from build123d import *

# Parameters (mm, degrees)
BOSS_EXTRU_1_DEPTH      = 10
ESQUISSE2_W             = 42
ESQUISSE2_H             = 42
BOSS_EXTRU_2_DEPTH      = 10
ESQUISSE3_W             = 42
ESQUISSE3_H             = 42
BOSS_EXTRU_3_DEPTH      = 10
ESQUISSE4_R             = 11
BOSS_EXTRU_4_DEPTH      = 3
CONG_1_R                = 0.5
ESQUISSE5_R             = 5
ENL_V_MAT_EXTRU_1_DEPTH = 10
ESQUISSE6_R             = 2.5
BOSS_EXTRU_5_DEPTH      = 30
ENL_V_MAT_EXTRU_2_DEPTH = 20
CHANFREIN1_SIZE         = 0.5
ESQUISSE8_R             = 1.5
ENL_V_MAT_EXTRU_3_DEPTH = 5
ENL_V_MAT_EXTRU_5_DEPTH = 41
ESQUISSE11_W            = 5
ESQUISSE11_H            = 10
ENL_V_MAT_EXTRU_6_DEPTH = 3


with BuildPart() as part:
    # Esquisse1 → Boss.-Extru.1 (new body, symmetric)
    with BuildSketch(Plane(origin=(0, 0, 0), x_dir=(0, 0, -1), z_dir=(1, 0, 0))):
        Polygon((6, 0), (36, 0), (42, -6), (42, -36), (36, -42), (6, -42), (0, -36), (0, -6), align=None)
    extrude(amount=BOSS_EXTRU_1_DEPTH, both=True)

    # Esquisse2 → Boss.-Extru.2 (add)
    with BuildSketch(Plane(origin=(10, 0, 0), x_dir=(0, 0, -1), z_dir=(1, 0, 0))):
        with Locations((21, -21)):
            Rectangle(ESQUISSE2_W, ESQUISSE2_H)
    extrude(amount=BOSS_EXTRU_2_DEPTH)

    # Esquisse3 → Boss.-Extru.3 (add)
    with BuildSketch(Plane.ZY.offset(10)):
        with Locations((-21, -21)):
            Rectangle(ESQUISSE3_W, ESQUISSE3_H)
    extrude(amount=BOSS_EXTRU_3_DEPTH)

    # Esquisse4 → Boss.-Extru.4 (add)
    with BuildSketch(Plane(origin=(20, 0, 0), x_dir=(0, 0, -1), z_dir=(1, 0, 0))):
        with Locations((21, -21)):
            Circle(ESQUISSE4_R)
    extrude(amount=BOSS_EXTRU_4_DEPTH)

    # Congé1
    cong_1_edges = [part.edges().sort_by_distance(p)[0] for p in [
        (20, -21, -10),
    ]]
    fillet(cong_1_edges, radius=CONG_1_R)

    # Esquisse5 → Enlèv. mat.-Extru.1 (cut)
    with BuildSketch(Plane(origin=(23, 0, 0), x_dir=(0, 0, -1), z_dir=(1, 0, 0))):
        with Locations((21, -21)):
            Circle(ESQUISSE5_R)
    extrude(amount=-ENL_V_MAT_EXTRU_1_DEPTH, mode=Mode.SUBTRACT)

    # Esquisse6 → Boss.-Extru.5 (add)
    with BuildSketch(Plane(origin=(13, 0, 0), x_dir=(0, 0, -1), z_dir=(1, 0, 0))):
        with Locations((21, -21)):
            Circle(ESQUISSE6_R)
    extrude(amount=BOSS_EXTRU_5_DEPTH)

    # Esquisse7 → Enlèv. mat.-Extru.2 (cut)
    with BuildSketch(Plane(origin=(43, 0, 0), x_dir=(0, 0, -1), z_dir=(1, 0, 0))):
        with BuildLine():
            Line((18.853641827, -19.718147202), (23.146358173, -19.718147202))
            ThreePointArc((23.146358173, -19.718147202), (21, -18.5), (18.853641827, -19.718147202))
        make_face()
    extrude(amount=-ENL_V_MAT_EXTRU_2_DEPTH, mode=Mode.SUBTRACT)

    # Chanfrein1
    chanfrein1_edges = [part.edges().sort_by_distance(p)[0] for p in [
        (43, -23.409968406, -20.335129874),
    ]]
    chamfer(chanfrein1_edges, length=CHANFREIN1_SIZE)

    # Esquisse8 → Enlèv. mat.-Extru.3 (cut)
    with BuildSketch(Plane(origin=(20, 0, 0), x_dir=(0, 0, -1), z_dir=(1, 0, 0))):
        with Locations((5, -5)):
            Circle(ESQUISSE8_R)
        with Locations((37, -5)):
            Circle(ESQUISSE8_R)
        with Locations((5, -37)):
            Circle(ESQUISSE8_R)
        with Locations((37, -37)):
            Circle(ESQUISSE8_R)
    extrude(amount=-ENL_V_MAT_EXTRU_3_DEPTH, mode=Mode.SUBTRACT)

    # Esquisse9 → Enlèv. mat.-Extru.5 (cut, through all)
    with BuildSketch(Plane(origin=(20, 0, 0), x_dir=(0, 0, -1), z_dir=(1, 0, 0))):
        Polygon((3, 0), (0, -3), (0, 0), align=None)
        Polygon((39, 0), (42, -3), (42, 0), align=None)
        Polygon((3, -42), (0, -39), (0, -42), align=None)
        Polygon((39, -42), (42, -39), (42, -42), align=None)
    extrude(amount=-ENL_V_MAT_EXTRU_5_DEPTH, mode=Mode.SUBTRACT)

    # Esquisse11 → Enlèv. mat.-Extru.6 (cut)
    with BuildSketch(Plane(origin=(0, 0, 0), x_dir=(1, 0, 0), z_dir=(0, 1, 0))):
        with Locations((-7.5, 21)):
            Rectangle(ESQUISSE11_W, ESQUISSE11_H)
    extrude(amount=-ENL_V_MAT_EXTRU_6_DEPTH, mode=Mode.SUBTRACT)


solid = part.part
Model file for the job. Use its own axes, mm. A direction names the side the tool comes from. Give positions to 0.01 mm unless a question says otherwise; leave off trailing zeros. Order: outer loops, then holes, each group sorted by start corner. A loop starts at its lowest first (then second) coordinate and runs counter-clockwise, first axis right, second up. Notation, with made-up numbers: M 2,50 L 15,50 A17 cw 15,60 Z; hole C 48.5,5.5 d8. An arc over 180 degrees is marked long. Write item = value, one per line.
Q1. Cut at A-A, the plane x = 17. List the corners of the cut face in (y, z), then the cut area to 3 significant figures.
Derived:
outline = M -42,-39 L -39,-42 L -3,-42 L 0,-39 L 0,-3 L -3,0 L -39,0 L -42,-3 Z; C -21,-21 d5; hole C -37,-37 d3; hole C -37,-5 d3; hole C -21,-21 d10; hole C -5,-37 d3; hole C -5,-5 d3
area = 1,660 mm2
Q2. Cut at D-D, the plane x = 36. List the corners of the cut face in (y, z).
Derived:
outline = M -19.72,-23.15 L -19.72,-18.85 A2.5 ccw long Z
Q3. Two-plate mould, pull along Y, no slides. Class faces 1 (the flat face through (-10, -40, -2)), 2 (the flat face through (0, 0, -21)), 3 (the cylindrical face through (27.54, -23.44, -20.46)): pulls with the +Y half, pulls with the -Y half, needs draft (parallel to the pull), parting line crosses it, or undercut.
Derived:
face_1 = needs draft
face_2 = pulls with the +Y half
face_3 = undercut
Q4. Cut at B-B, the plane y = -37. List the corners of the cut face in (x, z).
Derived:
outline = M -20,-42 L -10,-42 L -10,-41 L 10,-41 L 10,-42 L 20,-42 L 20,-38.5 L 15,-38.5 L 15,-35.5 L 20,-35.5 L 20,-6.5 L 15,-6.5 L 15,-3.5 L 20,-3.5 L 20,0 L 10,0 L 10,-1 L -10,-1 L -10,0 L -20,0 Z
Q5. Flat gauge pins, fed straight in: pin 1 (2.5 mm diameter, centred on x = -8.5, z = -23, fed in from +Y); pin 2 (0.9 mm diameter, centred on y = -4.5, z = -37.5, fed in from +X); pin 3 (12 mm diameter, centred on x = 10.5, y = -21, fed in from +Z); pin 4 (0.6 mm diameter, centred on y = -19, z = -21, fed in from +X). Where does each tip first touch, or does it go through?
Derived:
pin_1 = -3
pin_2 = 15
pin_3 = 0
pin_4 = 23
Q6. Tool access for faces 4 (the flat face through (10, -40, -2)), 5 (the flat face through (15, -5, -37)), 6 (the flat face through (0, -39, -39)): list every direction of +Z, -Z, +X, -X, +Y, -Y with a clear straight run to the whole face (end or side of a thin tool).
Derived:
face_4 = +Z, -Y
face_5 = +X
face_6 = -Z, -Y
Q7. Cut at C-C, the plane z = -21. List the corners of the cut face in (x, y).
Derived:
outline = M -20,-42 L 20,-42 L 20,-32.5 A0.5 cw 20.5,-32 L 23,-32 L 23,-26 L 13,-26 L 13,-23.5 L 42.5,-23.5 L 43,-23 L 43,-19.72 L 23,-19.72 L 23,-18.5 L 13,-18.5 L 13,-16 L 23,-16 L 23,-10 L 20.5,-10 A0.5 cw 20,-9.5 L 20,0 L -5,0 L -5,-3 L -10,-3 L -10,0 L -20,0 Z
Q8. Drill centre lines: line 1 (Y direction, x = 16.9, z = -5); line 2 (Z direction, x = 17.5, y = -4.5); line 3 (X direction, y = -10, z = -36). Where is each one in solid material? Low to high. Write a range as [from, to].
Derived:
line_1 = [-42, -38.5], [-35.5, -6.5], [-3.5, 0]
line_2 = [-42, -38.41], [-35.59, -6.41], [-3.59, 0]
line_3 = [-20, 20]
